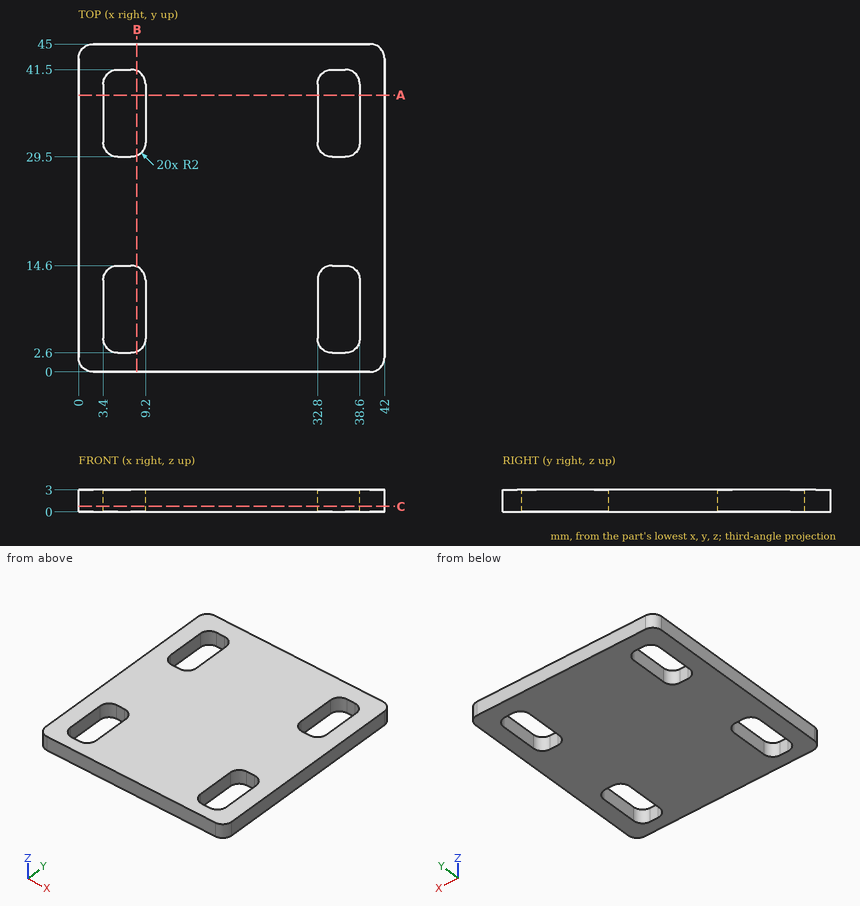
Can you work these out from the drawing? Everything is in mm from the part's minimum corner. Give positions to 0.01 mm unless a question says otherwise; leave off trailing zeros. Order: outer loops, then holes, each group sorted by start corner. A loop starts at its lowest first (then second) coordinate and runs counter-clockwise, first axis right, second up.
1. Suppose I cut it at A-A (y = 38). List the corners of the cut face in (x, z) for me.
2. Suppose I cut it at C-C (z = 0.75). Give the number of separate pieces and of enclosed holes in the cut face, plus the area to 3 significant figures.
3. Suppose I cut it at B-B (x = 8). List the corners of the cut face in (y, z) for me.
4. I need wall thicknesses on L1, parallel to Y at x = 35, z = 1.3; L2, parallel to X at y = 6, z = 1.6; L3, parallel to Y at x = 33, z = 0.65. Which ranges of each line are inside material? Lowest first, please.
Solved:
1. outline: (0, 0) - (3.4, 0) - (3.4, 3) - (0, 3) - close; (9.2, 0) - (32.8, 0) - (32.8, 3) - (9.2, 3) - close; (38.6, 0) - (42, 0) - (42, 3) - (38.6, 3) - close
2. separate pieces: 1
2. enclosed holes: 4
2. area: 1,620 mm2
3. outline: (0, 0) - (2.77, 0) - (2.77, 3) - (0, 3) - close; (14.43, 0) - (29.67, 0) - (29.67, 3) - (14.43, 3) - close; (41.33, 0) - (45, 0) - (45, 3) - (41.33, 3) - close
4. L1: y = 0 to 2.6, 14.6 to 29.5, 41.5 to 45
4. L2: x = 0 to 3.4, 9.2 to 32.8, 38.6 to 42
4. L3: y = 0 to 3.73, 13.47 to 30.63, 40.37 to 45
